Work out the finished part from the listing and answer in its coordinate system (mm). Face numbers are marked on the shaded views. A direction names the side the tool comes from. Coordinates: 2 decimals unless noted, no trailing zeros. Order: outer loops, then holes, each group sorted by start corner. A loop starts at its lowest first (then second) coordinate and runs counter-clockwise, first axis right, second up.
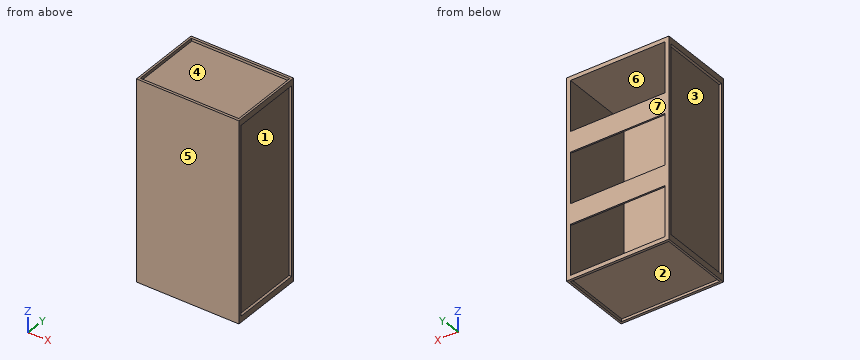
Autodesk Inventor part; units mm, degrees
ref_plane "YZ Plane" through (0, 0, 0) normal (1, 0, 0) x (0, 1, 0)
ref_plane "XZ Plane" through (0, 0, 0) normal (0, 1, 0) x (-1, 0, 0)
ref_plane "XY Plane" through (0, 0, 0) normal (0, 0, 1) x (1, 0, 0)
sketch "Sketch1" plane through (0, 0, 0) normal (0, 1, 0) x (-1, 0, 0)
  line L0 (-609.6, -1219.2) -> (609.6, -1219.2)
  line L1 (609.6, -1219.2) -> (609.6, 1219.2)
  line L2 (609.6, 1219.2) -> (-609.6, 1219.2)
  line L3 (-609.6, 1219.2) -> (-609.6, -1219.2)
  line L4 (-609.6, -1219.2) -> (609.6, 1219.2) construction
  line L5 (609.6, -1219.2) -> (-609.6, 1219.2) construction
  point P0 (0, 0)
  dimension "d0" = 1219.2
  dimension "d1" = 2438.4
extrude "Extrusion1" add sketch "Sketch1" along normal blind 914.4
sketch "Sketch2" plane through (0, 914.4, 0) normal (0, 1, 0) x (1, 0, 0)
  line L0 (590.55, 1200.15) -> (-590.55, 1200.15)
  line L1 (-590.55, 1200.15) -> (-590.55, -1200.15)
  line L2 (-590.55, -1200.15) -> (590.55, -1200.15)
  line L3 (590.55, -1200.15) -> (590.55, 1200.15)
  line L4 (590.55, 1200.15) -> (-590.55, -1200.15) construction
  line L5 (-590.55, 1200.15) -> (590.55, -1200.15) construction
  point P0 (0, 0)
  dimension "d4" = 1181.1
  dimension "d5" = 2400.3
extrude "Extrusion2" cut sketch "Sketch2" against normal blind 895.35
sketch "Sketch3" plane through (0, 914.4, 0) normal (0, 1, 0) x (1, 0, 0)
  line L0 (641.35, 1250.95) -> (-641.35, 1250.95)
  line L1 (-641.35, 1250.95) -> (-641.35, -1250.95)
  line L2 (-641.35, -1250.95) -> (641.35, -1250.95)
  line L3 (641.35, -1250.95) -> (641.35, 1250.95)
  line L4 (641.35, 1250.95) -> (-641.35, -1250.95) construction
  line L5 (-641.35, 1250.95) -> (641.35, -1250.95) construction
  line L6 (-590.55, -1200.15) -> (-590.55, 1200.15)
  line L7 (590.55, 1200.15) -> (-590.55, 1200.15)
  line L8 (-590.55, 1200.15) -> (-590.55, -1200.15)
  line L9 (-590.55, -1200.15) -> (590.55, -1200.15)
  line L10 (590.55, -1200.15) -> (590.55, 1200.15)
  line L11 (590.55, 1200.15) -> (-590.55, -1200.15) construction
  line L12 (-590.55, 1200.15) -> (590.55, -1200.15) construction
  point P0 (0, 0)
  point P1 (-590.55, 1200.15)
  dimension "d8" = 1282.7
  dimension "d9" = 2501.9
extrude "Extrusion3" add sketch "Sketch3" along normal blind 31.75
pattern_linear "Rectangular Pattern1" count 2 spacing 914.4 along (0, -1, 0) of "Extrusion3"
sketch "Sketch4" plane through (-641.35, 31.75, 1250.95) normal (0, 1, 0) x (1, 0, 0)
  line L0 (0, 0) -> (1282.7, 0)
  line L1 (1282.7, 0) -> (1282.7, 76.2)
  line L2 (1282.7, 0) -> (1282.7, 2501.9)
  line L3 (1282.7, 76.2) -> (1231.9, 76.2)
  line L4 (1231.9, 2451.1) -> (1231.9, 50.8)
  line L5 (1231.9, 76.2) -> (1231.9, 50.8)
  line L6 (1231.9, 50.8) -> (1257.3, 50.8)
  line L7 (1231.9, 50.8) -> (50.8, 50.8)
  line L8 (1257.3, 50.8) -> (1257.3, 0)
  line L9 (1257.3, 0) -> (1282.7, 0)
  point P0 (641.35, 1250.95)
  point P1 (1257.3, 0)
  dimension "d15" = 76.2
  dimension "d16" = 50.8
  dimension "d17" = 25.4
  dimension "d23" = 25.4
  dimension "d24" = 50.8
  dimension "d25" = 25.4
extrude "Extrusion4" add sketch "Sketch4" along normal blind 889
mirror "Mirror2" about plane through (0, 0, 0) normal (1, 0, 0) of "Extrusion4"
mirror "Mirror3" about plane through (0, 0, 0) normal (0, 0, 1) of "Extrusion4", "Mirror2"
sketch "Sketch5" plane through (0, 946.15, 0) normal (0, 1, 0) x (1, 0, 0)
  line L0 (-590.55, -1200.15) -> (-590.55, 1200.15)
  line L1 (590.55, -571.5) -> (-590.55, -571.5)
  line L2 (-590.55, -571.5) -> (-590.55, -317.5)
  line L3 (-590.55, -317.5) -> (590.55, -317.5)
  line L4 (590.55, -317.5) -> (590.55, -571.5)
  line L5 (590.55, -571.5) -> (-590.55, -317.5) construction
  line L6 (-590.55, -571.5) -> (590.55, -317.5) construction
  line L7 (590.55, 571.5) -> (-590.55, 571.5)
  line L8 (-590.55, 571.5) -> (-590.55, 317.5)
  line L9 (-590.55, 317.5) -> (590.55, 317.5)
  line L10 (590.55, 317.5) -> (590.55, 571.5)
  line L11 (590.55, 571.5) -> (-590.55, 317.5) construction
  line L12 (-590.55, 571.5) -> (590.55, 317.5) construction
  line L13 (-590.55, 1200.15) -> (590.55, 1200.15)
  line L14 (590.55, -1200.15) -> (-590.55, -1200.15)
  point P0 (0, 0)
  point P1 (0, -444.5)
  point P2 (0, 444.5)
  point P3 (-590.55, 63.5)
  point P4 (-590.55, 571.5)
  dimension "d26" = 254
  dimension "d27" = 254
  dimension "d31" = 628.65
  dimension "d34" = 628.65
  dimension "d35" = 635
extrude "Extrusion5" add sketch "Sketch5" against normal blind 19.05
properties part number "GlassCagesTank"
1. The part is cut by section A-A (x = 252). Determine the outline of the cut face in (y, z).
2. Consider probe 1 along Z at (x, y) = (-469.5, 540); probe 2 along Y at (x, z) = (-27, 372); probe 3 along X at (y, z) = (734.5, 154.5). Determine where each line is inside the solid, lowest interval first.
3. Flat-ended cylindrical pins translate along their axes: pin 1 (8 mm diameter, centred on y = 741, z = -580, fed in from -X); pin 2 (8 mm diameter, centred on x = -7.5, y = 141.5, fed in from +Z); pin 3 (6 mm diameter, centred on y = 704, z = 514.5, fed in from +X). Find the tip coordinate at first contact, or state that the pin passes through.
4. The mould has two halves that part along Y. Classify the marked faces 4, 5, 6 and 7: released by +Y, released by -Y, zero draft, split by the parting line, or undercut.
5. The part is cut by section D-D (z = 113). Determine the outline of the cut face in (x, y), plus the area to 3 significant figures.
6. The part is cut by section B-B (z = -432). Determine the outline of the cut face in (x, y), plus the area to 3 significant figures.
7. For the marked faces 1, 2 and 3, determine the directions among +Z, -Z, +X, -X, +Y, -Y from which every point of the face is accessible in a straight line to the end or side of a thin tool.
Worked out:
1. outline: (0, -1250.95) - (31.75, -1250.95) - (31.75, -1219.2) - (914.4, -1219.2) - (914.4, -1250.95) - (946.15, -1250.95) - (946.15, -1200.15) - (19.05, -1200.15) - (19.05, 1200.15) - (946.15, 1200.15) - (946.15, 1250.95) - (914.4, 1250.95) - (914.4, 1219.2) - (31.75, 1219.2) - (31.75, 1250.95) - (0, 1250.95) - close; (927.1, -571.5) - (946.15, -571.5) - (946.15, -317.5) - (927.1, -317.5) - close; (927.1, 317.5) - (946.15, 317.5) - (946.15, 571.5) - (927.1, 571.5) - close
2. probe 1: z = -1219.2 to -1200.15, 1200.15 to 1219.2
2. probe 2: y = 0 to 19.05, 927.1 to 946.15
2. probe 3: x = -609.6 to -590.55, 590.55 to 609.6
3. pin 1: stops at x = -609.6
3. pin 2: stops at z = 1219.2
3. pin 3: stops at x = 609.6
4. face 4: undercut
4. face 5: released by -Y
4. face 6: zero draft
4. face 7: released by +Y
5. outline: (-641.35, 0) - (641.35, 0) - (641.35, 31.75) - (609.6, 31.75) - (609.6, 914.4) - (641.35, 914.4) - (641.35, 946.15) - (590.55, 946.15) - (590.55, 19.05) - (-590.55, 19.05) - (-590.55, 946.15) - (-641.35, 946.15) - (-641.35, 914.4) - (-609.6, 914.4) - (-609.6, 31.75) - (-641.35, 31.75) - close
5. area: 62,600 mm2
6. outline: (-641.35, 0) - (641.35, 0) - (641.35, 31.75) - (609.6, 31.75) - (609.6, 914.4) - (641.35, 914.4) - (641.35, 946.15) - (-641.35, 946.15) - (-641.35, 914.4) - (-609.6, 914.4) - (-609.6, 31.75) - (-641.35, 31.75) - close; hole (-590.55, 19.05) - (590.55, 19.05) - (590.55, 927.1) - (-590.55, 927.1) - close
6. area: 85,100 mm2
7. face 1: +X
7. face 2: -Z
7. face 3: -X
